Read the model definition and answer for the solid it produces. Units are mm, in the model's axes. A direction names the side the tool comes from. Coordinates: 2 decimals unless noted, no trailing zeros. Loops run counter-clockwise (first coordinate to the right, second up) from the corner with the lowest first, then second, coordinate; pieces in that order, holes last.
from build123d import *

# Parameters (mm, degrees)
SKETCH1_W                    = 60
SKETCH1_H                    = 30
BASE_FLANGE1_DEPTH           = 0.635
SKETCH9_W                    = 24.6
SKETCH9_H                    = 12
CUT_EXTRUDE1_DEPTH           = 34.547030047
CUT_EXTRUDE2_DEPTH           = 34.547030047
EDGE_FLANGE1_STRIP_W         = 4.54
EDGE_FLANGE1_STRIP_H         = 0.635
EDGE_FLANGE1_STRIP_CUT_DEPTH = 30
EDGE_FLANGE1_DEPTH           = 30
SKETCH14_R                   = 2.65
CUT_EXTRUDE3_DEPTH           = 63.276532097
FILLET1_R                    = 2


# Sheet-metal steps are written as plain solids
with BuildPart() as part:
    # Sketch1 → Base-Flange1 (new body)
    with BuildSketch(Plane(origin=(0, 0, 0), x_dir=(0, 0, -1), z_dir=(1, 0, 0))):
        Rectangle(SKETCH1_W, SKETCH1_H)
    extrude(amount=-BASE_FLANGE1_DEPTH)

    # Sketch9 → Cut-Extrude1 (cut, through all)
    with BuildSketch(Plane(origin=(0, 0, 0), x_dir=(0, 0, -1), z_dir=(1, 0, 0))):
        with Locations((-5.35, 0)):
            Rectangle(SKETCH9_W, SKETCH9_H)
    extrude(amount=-CUT_EXTRUDE1_DEPTH, mode=Mode.SUBTRACT)

    # Sketch10 → Cut-Extrude2 (cut, through all)
    with BuildSketch(Plane.ZY.offset(0.635)):
        with BuildLine():
            Line((-9.3, 1.15), (-7.3, 1.15))
            ThreePointArc((-7.3, 1.15), (-6.15, 0), (-7.3, -1.15))
            Line((-7.3, -1.15), (-9.3, -1.15))
            ThreePointArc((-9.3, -1.15), (-10.45, 0), (-9.3, 1.15))
        make_face()
        with BuildLine():
            Line((18, 1.15), (20, 1.15))
            ThreePointArc((20, 1.15), (21.15, 0), (20, -1.15))
            Line((20, -1.15), (18, -1.15))
            ThreePointArc((18, -1.15), (16.85, 0), (18, 1.15))
        make_face()
    extrude(amount=-CUT_EXTRUDE2_DEPTH, mode=Mode.SUBTRACT)

    # Edge-Flange1 strip (across the edge) → Edge-Flange1 strip cut (cut)
    with BuildSketch(Plane(origin=(0, 15, 30), x_dir=(0, 0, -1), z_dir=(0, -1, 0))):
        with Locations((-0.635, -0.3175)):
            Rectangle(EDGE_FLANGE1_STRIP_W, EDGE_FLANGE1_STRIP_H)
    extrude(amount=EDGE_FLANGE1_STRIP_CUT_DEPTH, mode=Mode.SUBTRACT)

    # Edge-Flange1 section (across the edge) → Edge-Flange1 (add)
    with BuildSketch(Plane(origin=(0, 15, 30), x_dir=(0, 0, -1), z_dir=(0, -1, 0))):
        with BuildLine():
            Line((0, 1), (0, 11.365))
            Line((0, 11.365), (0.635, 11.365))
            Line((0.635, 11.365), (0.635, 1))
            ThreePointArc((0.635, 1), (0.927893219, 0.292893219), (1.635, 0))
            Line((1.635, 0), (1.635, -0.635))
            ThreePointArc((1.635, -0.635), (0.478880413, -0.156119587), (0, 1))
        make_face()
    extrude(amount=EDGE_FLANGE1_DEPTH)

    # Sketch14 → Cut-Extrude3 (cut, through all)
    with BuildSketch(Plane(origin=(0, 0, 29.365), x_dir=(-1, 0, 0), z_dir=(0, 0, -1))):
        with Locations((-6.1825, -8)):
            Circle(SKETCH14_R)
        with BuildLine():
            Line((-8.8325, 4.5), (-8.8325, 9.5))
            ThreePointArc((-8.8325, 9.5), (-6.1825, 12.15), (-3.5325, 9.5))
            Line((-3.5325, 9.5), (-3.5325, 4.5))
            ThreePointArc((-3.5325, 4.5), (-6.1825, 1.85), (-8.8325, 4.5))
        make_face()
    extrude(amount=-CUT_EXTRUDE3_DEPTH, mode=Mode.SUBTRACT)

    # Fillet1
    fillet1_edges = [part.edges().sort_by_distance(p)[0] for p in [
        (11.365, 15, 29.6825),
        (11.365, -15, 29.6825),
        (-0.3175, -15, -30),
        (-0.3175, 15, -30),
    ]]
    fillet(fillet1_edges, radius=FILLET1_R)


solid = part.part
Q1. A cutting plane is placed at C-C (x = 4.25). Give the vertices of the cut face in (y, z) (3 decimals).
Findings below:
outline: (-15, 29.365) - (-9.813, 29.365) - (-9.813, 30) - (-15, 30) - close; (-6.187, 29.365) - (2.687, 29.365) - (2.687, 30) - (-6.187, 30) - close; (11.313, 29.365) - (15, 29.365) - (15, 30) - (11.313, 30) - close
Q2. A cutting plane is placed at D-D (y = 2.5). Give the vertices of the cut face in (x, z) (3 decimals), then the cut area to 3 significant figures.
Findings below:
outline: (-0.635, -30) - (0, -30) - (0, -6.95) - (-0.635, -6.95) - close; (-0.635, 17.65) - (0, 17.65) - (0, 28.365) arc R1 cw to (1, 29.365) - (4.444, 29.365) - (4.444, 30) - (1, 30) arc R1.635 ccw to (-0.635, 28.365) - close; (7.921, 29.365) - (11.365, 29.365) - (11.365, 30) - (7.921, 30) - close
area: 27.1 mm2
Q3. A cutting plane is placed at B-B (z = 14.5). Give the vertices of the cut face in (x, y) (3 decimals), then the cut area to 3 significant figures.
Findings below:
outline: (-0.635, -15) - (0, -15) - (0, -6) - (-0.635, -6) - close; (-0.635, 6) - (0, 6) - (0, 15) - (-0.635, 15) - close
area: 11.4 mm2
Q4. Flat-ended cylindrical pins translate along their axes: pin 1 Ø0.5 at (x, y) = (0, -3) entering from +Z; pin 2 Ø0.7 at (x, y) = (-0.5, 3) entering from +Z; pin 3 Ø9 at (y, z) = (1.5, -10) entering from +X. Find the tip coordinate at first contact, or state that the pin passes through.
Findings below:
pin 1: stops at z = 29.82
pin 2: stops at z = 29.53
pin 3: stops at x = 0
Q5. Determine the mould class of faces 5 (the face through (-0.32, -0.03, -10.45)), 6 (the face through (4.96, -10.35, 29.68)), 7 (the face through (6.24, 12.15, 29.68)), 8 (the face through (-0.635, 7, 0)) for opening direction X: +X half, -X half, draft (parallel to the pull), parting line (faces both ways), or undercut.
Findings below:
face 5: draft
face 6: undercut
face 7: undercut
face 8: -X half
Q6. Which of the six approach directions +Z, -Z, +X, -X, +Y, -Y give full straight-line access (tool end or side, diameter ignored) to faces 1 (the face through (6, 0, 29.365)), 2 (the face through (6.12, 1.85, 29.68)), 3 (the face through (-0.32, -14.43, -29.4)), 4 (the face through (-0.32, 0.03, 21.15))?
Findings below:
face 1: -Z, +X, +Y, -Y
face 2: +Z, -Z
face 3: -Z, +X, -X, -Y
face 4: +X, -X
Q7. Straight lines are drawn through the part: probe 1 along Z at (x, y) = (9.25, 13) (3 decimals); probe 2 along X at (y, z) = (-12, 27) (3 decimals); probe 3 along Z at (x, y) = (0.25, 4). For each, find the intervals that lie inside material, in ascending order.
Findings below:
probe 1: z = 29.365 to 30
probe 2: x = -0.635 to 0
probe 3: z = 29.03 to 29.82
Q8. A cutting plane is placed at A-A (y = -8). Give the vertices of the cut face in (x, z) (1 decimal).
Findings below:
outline: (-0.6, -30) - (0, -30) - (0, 28.4) arc R1 cw to (1, 29.4) - (3.5, 29.4) - (3.5, 30) - (1, 30) arc R1.6 ccw to (-0.6, 28.4) - close; (8.8, 29.4) - (11.4, 29.4) - (11.4, 30) - (8.8, 30) - close
